Verification items for this drawing (mm, ordinates from the low corner). A direction names the side the tool comes from. Coordinates: 2 decimals unless noted, no trailing zeros. Write each loop counter-clockwise with the first axis right and the second up, starting at its lowest first coordinate (ties: lowest second). Pieces come first, ordered by that corner, then holes. Notation, with made-up numbers: (26.5, 13) -> (70.5, 13) arc R36 ccw to (70.5, 48) -> close; hole circle Ø10 at (0.5, 15.25). An arc over 180 degrees is marked (long way). One line per question, with ' | ' between items.
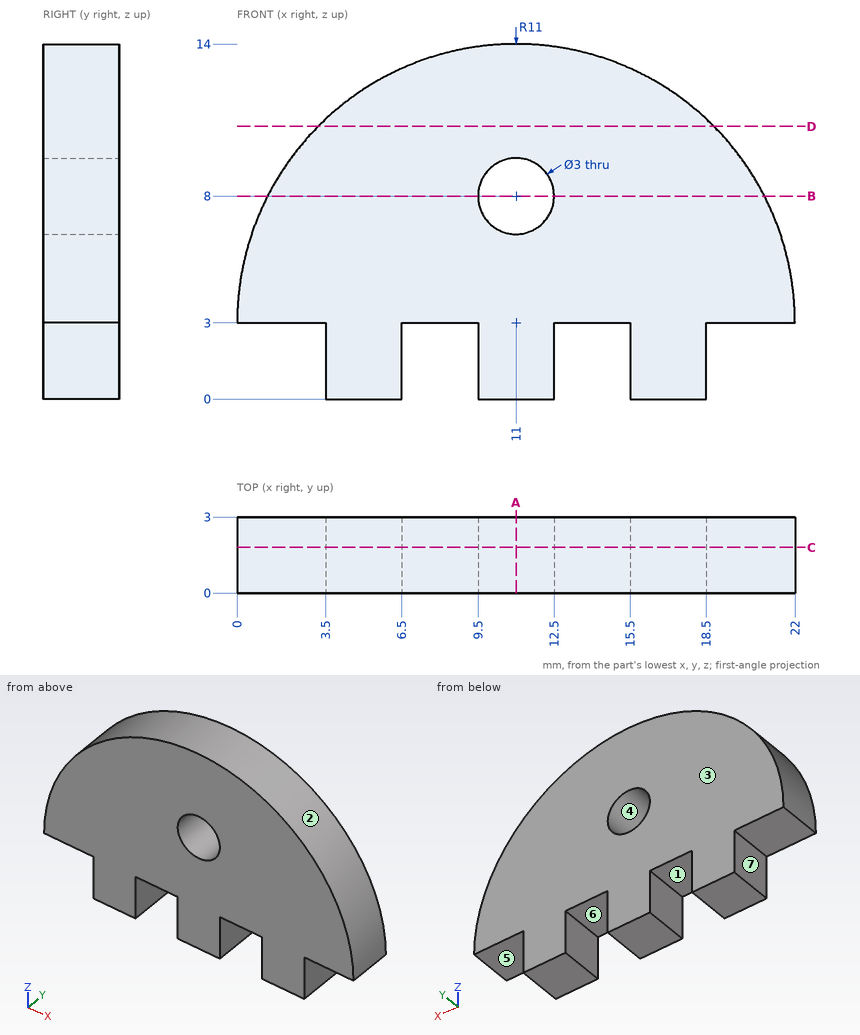
(1) Tool access check on the marked faces 4, 5, 6 and 7. Record the directions out of +Z, -Z, +X, -X, +Y, -Y that give a thin tool (end or side, any length) a straight path to the whole face; none if there is none.
Answers below:
face 4: +Y, -Y | face 5: -Z, +X, +Y, -Y | face 6: -Z, +Y, -Y | face 7: -Z, -X, +Y, -Y
(2) Material ranges on line 1 (Z direction, x = 11, y = 1.65); line 2 (Z direction, x = 12.25, y = 1.55); line 3 (X direction, y = 0.6, z = 7), recorded low to high.
Answers below:
line 1: z = 0 to 6.5, 9.5 to 14 | line 2: z = 0 to 7.17, 8.83 to 13.93 | line 3: x = 0.75 to 9.88, 12.12 to 21.25
(3) Draft check along X on the marked faces 1, 2 and 3. Enter one of: pulls with the +X half, pulls with the -X half, needs draft (parallel to the pull), parting line crosses it, or undercut.
Answers below:
face 1: undercut | face 2: parting line crosses it | face 3: needs draft
(4) Cross-section at C-C (y = 1.8). Record the cut outline in (x, z), plus the area to 3 significant figures.
Answers below:
outline: (0, 3) -> (3.5, 3) -> (3.5, 0) -> (6.5, 0) -> (6.5, 3) -> (9.5, 3) -> (9.5, 0) -> (12.5, 0) -> (12.5, 3) -> (15.5, 3) -> (15.5, 0) -> (18.5, 0) -> (18.5, 3) -> (22, 3) arc R11 ccw to start; hole circle Ø3 at (11, 8) | area: 210 mm²
(5) Cross-section at A-A (x = 11). Record the cut outline in (y, z), plus the area to 3 significant figures.
Answers below:
outline: (0, 0) -> (3, 0) -> (3, 6.5) -> (0, 6.5) -> close; (0, 9.5) -> (3, 9.5) -> (3, 14) -> (0, 14) -> close | area: 33.0 mm²
(6) Cross-section at B-B (z = 8). Record the cut outline in (x, y), plus the area to 3 significant figures.
Answers below:
outline: (1.2, 0) -> (9.5, 0) -> (9.5, 3) -> (1.2, 3) -> close; (12.5, 0) -> (20.8, 0) -> (20.8, 3) -> (12.5, 3) -> close | area: 49.8 mm²
(7) Cross-section at D-D (z = 10.75). Record the cut outline in (x, y).
Answers below:
outline: (3.19, 0) -> (18.81, 0) -> (18.81, 3) -> (3.19, 3) -> close
(8) Depth check by flat-ended pin: P1, Ø0.9, axis at x = 2.5, y = 1.5, coming from the -Z side; P2, Ø1.5, axis at y = 1.5, z = 1, coming from the +X side; P3, Ø0.9, axis at y = 2, z = 1.5, coming from the -X side. Enter the tip coordinate at first touch or a pass-through.
Answers below:
P1: stops at z = 3 | P2: stops at x = 18.5 | P3: stops at x = 3.5
